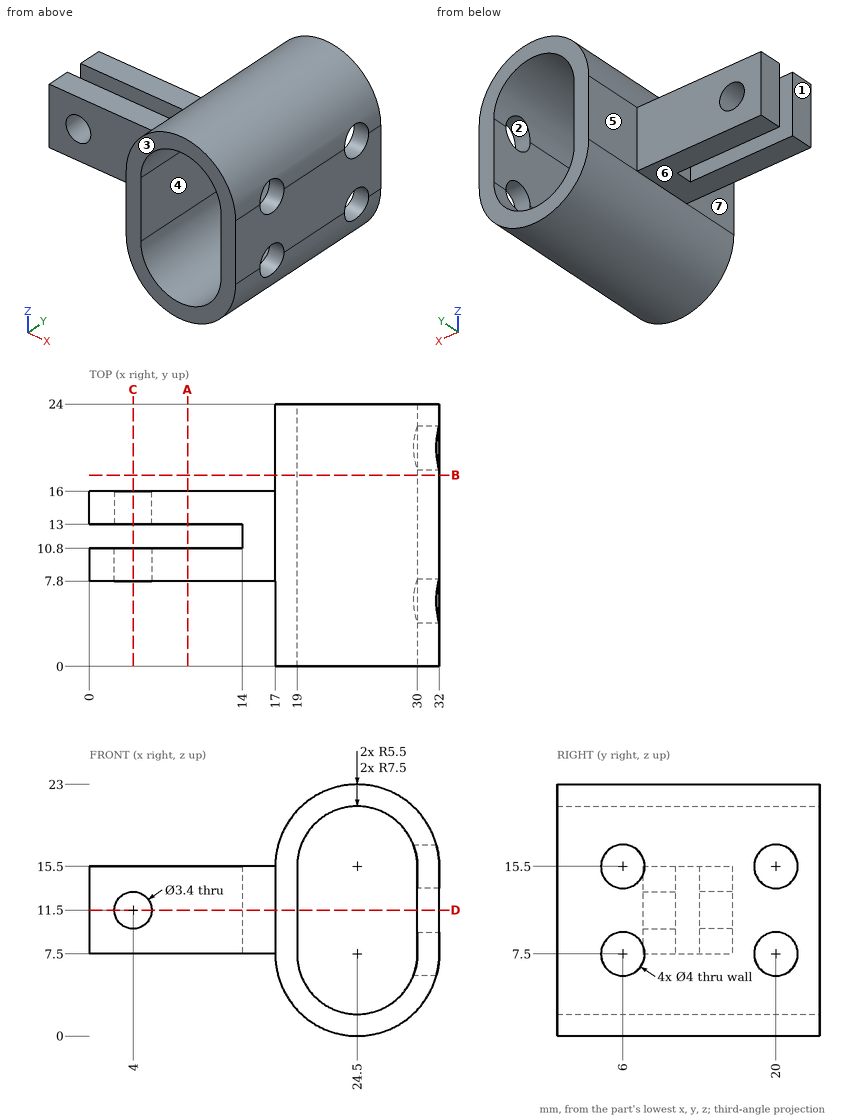
Design review of the part shown in the three views and the two pictorial views. Dimensions are in mm from the part's minimum x, y and z. A direction names the side the tool comes from. Give positions to 0.01 mm unless a question says otherwise; leave off trailing zeros. Write each loop counter-clockwise with the first axis right and the second up, starting at its lowest first coordinate (ties: lowest second). Pieces come first, ordered by that corner, then holes.
(1) Mouldability with a two-part tool opening along Y and no side actions: class the marked faces 1, 2 and 3 as +Y half, -Y half, draft (parallel to the pull), parting line (faces both ways), or undercut.
Checked values:
face 1: draft
face 2: undercut
face 3: -Y half
(2) Add section B-B (y = 17.5). Give the boundary of the cut face in (x, z), and give its area (3 significant figures).
Checked values:
outline: (17, 7.5) arc R7.5 ccw to (32, 7.5) - (32, 15.5) arc R7.5 ccw to (17, 15.5) - close; hole (19, 7.5) arc R5.5 ccw to (30, 7.5) - (30, 15.5) arc R5.5 ccw to (19, 15.5) - close
area: 114 mm2
(3) Add section D-D (z = 11.5). Give the boundary of the cut face in (x, y).
Checked values:
outline: (0, 7.8) - (2.3, 7.8) - (2.3, 10.8) - (0, 10.8) - close; (0, 13) - (2.3, 13) - (2.3, 16) - (0, 16) - close; (5.7, 7.8) - (17, 7.8) - (17, 0) - (19, 0) - (19, 24) - (17, 24) - (17, 16) - (5.7, 16) - (5.7, 13) - (14, 13) - (14, 10.8) - (5.7, 10.8) - close; (30, 0) - (32, 0) - (32, 24) - (30, 24) - close
(4) Clearance check with flat-ended pins moving along their axes: pin 1 Ø3 at (x, z) = (4, 11.5) entering from -Y; pin 2 Ø4 at (x, z) = (6, 10.5) entering from -Y; pin 3 Ø4 at (x, z) = (4, 11.5) entering from +Y; pin 4 Ø1.8 at (y, z) = (12, 9.5) entering from -X. State where each tip first meets the part, or that it passes through.
Checked values:
pin 1: passes through
pin 2: stops at y = 7.8
pin 3: stops at y = 16
pin 4: stops at x = 14
(5) Add section C-C (x = 4). Give the boundary of the cut face in (y, z), and give its area (3 significant figures).
Checked values:
outline: (7.8, 7.5) - (10.8, 7.5) - (10.8, 9.8) - (7.8, 9.8) - close; (7.8, 13.2) - (10.8, 13.2) - (10.8, 15.5) - (7.8, 15.5) - close; (13, 7.5) - (16, 7.5) - (16, 9.8) - (13, 9.8) - close; (13, 13.2) - (16, 13.2) - (16, 15.5) - (13, 15.5) - close
area: 27.6 mm2
(6) Tool access review of the marked faces 4, 5, 6 and 7: name each direction out of +Z, -Z, +X, -X, +Y, -Y from which nothing blocks a thin tool from reaching the whole face with its end or side.
Checked values:
face 4: +Y, -Y
face 5: +Z, -Z, -X, +Y
face 6: -Z, -X, +Y, -Y
face 7: +Z, -Z, -X, -Y
(7) Add section A-A (x = 9). Give the boundary of the cut face in (y, z).
Checked values:
outline: (7.8, 7.5) - (10.8, 7.5) - (10.8, 15.5) - (7.8, 15.5) - close; (13, 7.5) - (16, 7.5) - (16, 15.5) - (13, 15.5) - close
(8) Wall thickness on line 1 along X through (y, z) = (7.5, 13.25); line 2 along X through (y, z) = (14.25, 13.5); line 3 along Y through (x, z) = (3.5, 15): over which ranges is each line inside the solid? List them lowest first.
Checked values:
line 1: x = 17 to 19, 30 to 32
line 2: x = 0 to 19, 30 to 32
line 3: y = 7.8 to 10.8, 13 to 16
